Model file for the job. Use its own axes, mm. A direction names the side the tool comes from. Give positions to 0.01 mm unless a question says otherwise; leave off trailing zeros. Write each loop counter-clockwise with the first axis right and the second up, starting at its lowest first coordinate (ties: lowest second). Pieces come first, ordered by that corner, then holes.
```python
from build123d import *

# Parameters (mm, degrees)
SKETCH1_W               = 121.6
SKETCH1_H               = 61.004801574
BOSS_EXTRUDE1_DEPTH     = 3
SKETCH3_W               = 3
SKETCH3_H               = 8
BOSS_EXTRUDE2_DEPTH     = 3
SKETCH5_W               = 7
SKETCH5_H               = 3
CUT_EXTRUDE1_DEPTH      = 71.780198176
MIRROR3_COPY_1_SKETCH_W = 7
MIRROR3_COPY_1_SKETCH_H = 3
MIRROR3_COPY_1_DEPTH    = 71.780198176
VELCROHOLE_DEPTH        = 71.780198176
VELCROHOLE_DEPTH_BACK   = 71.780198176


with BuildPart() as part:
    # Sketch1 → Boss-Extrude1 (new body)
    with BuildSketch(Plane.XY):
        Rectangle(SKETCH1_W, SKETCH1_H)
    extrude(amount=BOSS_EXTRUDE1_DEPTH)

    # Sketch3 → Boss-Extrude2 (add)
    with BuildSketch(Plane(origin=(60.8, 0, 0), x_dir=(0, 0, -1), z_dir=(1, 0, 0))):
        with Locations((-1.5, 26.502400787)):
            Rectangle(SKETCH3_W, SKETCH3_H)
        with Locations((-1.5, 3.502400787)):
            Rectangle(SKETCH3_W, SKETCH3_H)
        with Locations((-1.5, -19.497599213)):
            Rectangle(SKETCH3_W, SKETCH3_H)
    boss_extrude2 = extrude(amount=BOSS_EXTRUDE2_DEPTH)

    # Mirror1: Boss-Extrude2 across plane
    add(boss_extrude2.mirror(Plane(origin=(0, 0, 0), x_dir=(0, 0, 1), z_dir=(1, 0, 0))))

    # Sketch5 → Cut-Extrude1 (cut, through all)
    with BuildSketch(Plane(origin=(0, 0, 0), x_dir=(-1, 0, 0), z_dir=(0, 0, -1))):
        with Locations((-57.3, 15.002400787)):
            Rectangle(SKETCH5_W, SKETCH5_H)
        Polygon((-53.8, 19.002400787), (-53.8, 16.502400787), (-53.8, 13.502400787), (-53.8, 11.002400787), (-51.8, 11.002400787), (-51.8, 19.002400787), align=None)
    cut_extrude1 = extrude(amount=-CUT_EXTRUDE1_DEPTH, mode=Mode.SUBTRACT)

    # Mirror2: Cut-Extrude1 across plane
    add(cut_extrude1.mirror(Plane(origin=(0, 0, 0), x_dir=(0, 0, 1), z_dir=(1, 0, 0))), mode=Mode.SUBTRACT)

    # Mirror3: Cut-Extrude1 across plane
    add(cut_extrude1.mirror(Plane(origin=(0, 3.502400787, 0), x_dir=(0, 0, 1), z_dir=(0, -1, 0))), mode=Mode.SUBTRACT)

    # Mirror3 copy 1 sketch → Mirror3 copy 1 (cut, through all)
    with BuildSketch(Plane(origin=(0, 7.004801574, 0), x_dir=(1, 0, 0), z_dir=(0, 0, -1))):
        with Locations((-57.3, 15.002400787)):
            Rectangle(MIRROR3_COPY_1_SKETCH_W, MIRROR3_COPY_1_SKETCH_H)
        Polygon((-53.8, 19.002400787), (-53.8, 16.502400787), (-53.8, 13.502400787), (-53.8, 11.002400787), (-51.8, 11.002400787), (-51.8, 19.002400787), align=None)
    extrude(amount=-MIRROR3_COPY_1_DEPTH, mode=Mode.SUBTRACT)

    # Sketch6 → VelcroHole (cut, two sides: drawn at the far end of the back side and taken through both)
    with BuildSketch(Plane(origin=(0, 0, 0), x_dir=(-1, 0, 0), z_dir=(0, 0, -1)).offset(-VELCROHOLE_DEPTH_BACK)):
        with BuildLine():
            Line((-23.721301338, -19.330337048), (23.721301338, -19.330337048))
            ThreePointArc((23.721301338, -19.330337048), (26.648610865, -22.257646575), (23.721301338, -25.184956102))
            Line((23.721301338, -25.184956102), (-23.721301338, -25.184956102))
            ThreePointArc((-23.721301338, -25.184956102), (-26.648610865, -22.257646575), (-23.721301338, -19.330337048))
        make_face()
    extrude(amount=VELCROHOLE_DEPTH + VELCROHOLE_DEPTH_BACK, mode=Mode.SUBTRACT)


solid = part.part
```
1. Slice it at A-A, the plane x = 20.5. Write the cut outline in (y, z).
Calculated:
outline: (-30.5, 0) - (-25.18, 0) - (-25.18, 3) - (-30.5, 3) - close; (-19.33, 0) - (30.5, 0) - (30.5, 3) - (-19.33, 3) - close
2. Probe probe 1 along Y at (x, z) = (-56, 1.45); probe 2 along Y at (x, z) = (20.5, 2.7); probe 3 along X at (y, z) = (10.5, 2.7). List the from-to ranges inside material, lowest first.
Calculated:
probe 1: y = -30.5 to -9.5, -6.5 to 13.5, 16.5 to 30.5
probe 2: y = -30.5 to -25.18, -19.33 to 30.5
probe 3: x = -60.8 to 60.8
3. Which spindle directions (+Z, -Z, +X, -X, +Y, -Y) get a long thin tool onto all of the face, cutting with end or side? Do faces 1 (the flat face through (-62, 7.502, 2)), 2 (the flat face through (51.8, -8, 1)), 3 (the flat face through (57, 16.502, 1)). Say none if no direction does.
Calculated:
face 1: +Z, -Z, -X
face 2: +Z, -Z
face 3: +Z, -Z, +X
4. Pin check, flat tips, straight feed: P1, Ø1.5, axis at y = -27.5, z = 1.5, coming from the -X side; P2, Ø0.8, axis at y = 12, z = 1, coming from the +X side. Stop position of each tip, or through.
Calculated:
P1: stops at x = -60.8
P2: stops at x = 60.8
5. Pull direction X, two halves, no side cores. Call faces 4 (the flat face through (63.8, 4, 2)), 5 (the flat face through (-62, -15.498, 2)), 6 (the flat face through (-60.8, -27, 1)), 7 (the flat face through (53.8, -11, 1)): +X half, -X half, draft (parallel to the pull), parting line (faces both ways), or undercut.
Calculated:
face 4: +X half
face 5: draft
face 6: -X half
face 7: undercut
